Check sheet for the modelled part. Datum: model origin and axes. Units: mm. Face numbers are marked on the shaded views. Round coordinates to 2 decimals unless told otherwise and drop trailing zeros. Loops run counter-clockwise (first coordinate to the right, second up) from the corner with the lowest first, then second, coordinate; pieces in that order, holes last. Notation, with made-up numbers: (6.25, 77) - (61.25, 77) arc R23 ccw to (61.25, 93) - close; hole circle Ø2 at (-14, 89). An arc over 180 degrees is marked (long way). Put each result on its own line as item: value. Start each with the question number.
Item 1: Material ranges on line 1 along Y through (x, z) = (-5, 18.25); line 2 along Y through (x, z) = (0.25, 23.5); line 3 along X through (y, z) = (0.1, 10.5), recorded low to high.
Item 2: Draft check along X on the marked faces 1, 2 and 3. Enter one of: pulls with the +X half, pulls with the -X half, needs draft (parallel to the pull), parting line crosses it, or undercut.
Item 3: Section check D-D, the plane x = 6.25. Record the cut outline in (y, z).
Item 4: Section check A-A, the plane y = 0.9. Record the cut outline in (x, z), and give its area (3 significant figures).
Item 5: Section check C-C, the plane x = -1. Record the cut outline in (y, z), and give its area (3 significant figures).
Item 6: Section check B-B, the plane z = 12.5. Record the cut outline in (x, y).
Item 7: Gauge pin test, flat end, axial feed: pin 1 Ø2 at (y, z) = (2, 2.5) entering from +X. Record the tip position at first contact, or that the pin passes through.
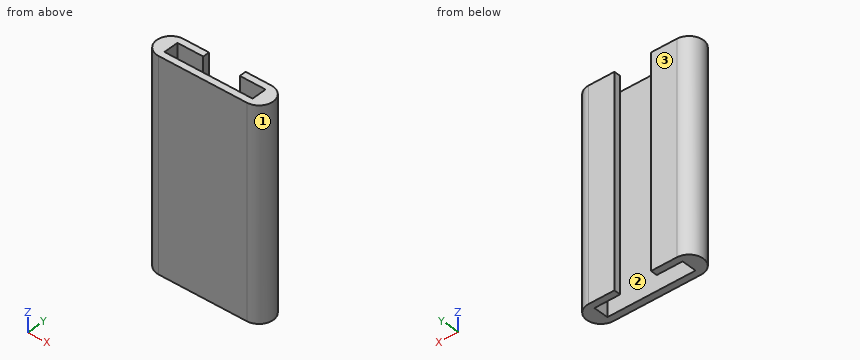
from build123d import *

# Parameters (mm, degrees)
F1_DEPTH = 25


with BuildPart() as f1:
    # F0 (on Top) → F1 (new body)
    with BuildSketch(Plane.XY):
        with BuildLine():
            Line((5.3, 0), (0, 0))
            Line((0, 0), (-5.3, 0))
            Line((-5.3, 0), (-5.3, 1.8))
            Line((-5.3, 1.8), (-2.2, 1.8))
            Line((-2.2, 1.8), (-2.2, 2.6))
            Line((-2.2, 2.6), (-5.3, 2.6))
            ThreePointArc((-5.3, 2.6), (-7, 0.9), (-5.3, -0.8))
            Line((-5.3, -0.8), (0, -0.8))
            Line((0, -0.8), (5.3, -0.8))
            ThreePointArc((5.3, -0.8), (7, 0.9), (5.3, 2.6))
            Line((5.3, 2.6), (2.2, 2.6))
            Line((2.2, 2.6), (2.2, 1.8))
            Line((2.2, 1.8), (5.3, 1.8))
            Line((5.3, 1.8), (5.3, 0))
        make_face()
    extrude(amount=F1_DEPTH)


solid = f1.part
Check result:
1. line 1: -0.8 to 0, 1.8 to 2.6
1. line 2: -0.8 to 0
1. line 3: -6.8 to -5.3, 5.3 to 6.8
2. face 1: pulls with the +X half
2. face 2: undercut
2. face 3: needs draft
3. outline: (-0.51, 0) - (2.31, 0) - (2.31, 25) - (-0.51, 25) - close
4. outline: (-7, 0) - (-5.3, 0) - (-5.3, 25) - (-7, 25) - close; (5.3, 0) - (7, 0) - (7, 25) - (5.3, 25) - close
4. area: 85.0 mm²
5. outline: (-0.8, 0) - (0, 0) - (0, 25) - (-0.8, 25) - close
5. area: 20.0 mm²
6. outline: (-5.3, -0.8) - (5.3, -0.8) arc R1.7 ccw to (5.3, 2.6) - (2.2, 2.6) - (2.2, 1.8) - (5.3, 1.8) - (5.3, 0) - (-5.3, 0) - (-5.3, 1.8) - (-2.2, 1.8) - (-2.2, 2.6) - (-5.3, 2.6) arc R1.7 ccw to start
7. pin 1: x = 7
